Autodesk Inventor part; units mm, degrees
ref_plane "YZ Plane" through (0, 0, 0) normal (1, 0, 0) x (0, 1, 0)
ref_plane "XZ Plane" through (0, 0, 0) normal (0, 1, 0) x (-1, 0, 0)
ref_plane "XY Plane" through (0, 0, 0) normal (0, 0, 1) x (1, 0, 0)
sketch "スケッチ1" plane through (0, 0, 0) normal (0, 0, 1) x (1, 0, 0)
  line L0 (-30, 18) -> (30, 18)
  line L1 (30, 18) -> (30, -18)
  line L2 (30, -18) -> (-30, -18)
  line L3 (-30, -18) -> (-30, 18)
  line L4 (0, 0) -> (0, 18) construction
  line L5 (0, 0) -> (30, 0) construction
  dimension "d0" = 36
  dimension "d1" = 60
extrude "プレート1" add sketch "スケッチ1" along normal blind 3
sketch "スケッチ13" plane through (0, 0, 0) normal (0, 0, -1) x (-1, 0, 0)
  line L0 (0, 0) -> (30, 0) construction
  line L1 (30, -18) -> (30, 18)
  line L2 (-30, 18) -> (-30, -18)
  point P0 (23, 0)
  point P1 (-7, 0)
  dimension "d127" = 30
  dimension "d129" = 7
hole "穴10" at (-23, 0, 0) at (7, 0, 0) direction (0, 0, 1) diameter 7.9 depth 3
sketch "スケッチ15" plane through (0, 0, 0) normal (0, 0, -1) x (-1, 0, 0)
  circle A0 centre (-40, 0) radius 21
  line L0 (-30, -18) -> (-30, 18)
  point P0 (0, 0)
  dimension "d130" = 42
  dimension "d131" = 10
extrude "押し出し1" add sketch "スケッチ15" against normal up to surface (3 mm away)
fillet "フィレット1" radius 10 2 edges at (-30, 18, 1.5) (-30, -18, 1.5)
sketch "スケッチ16" plane through (0, 0, 0) normal (0, 0, -1) x (-1, 0, 0)
  arc A0 (-29.1833, 18) -> (-29.1833, -18) centre (-40, 0) ccw
  circle A1 centre (-40, 0) radius 14.5
  point P0 (0, 0)
  dimension "d134" = 29
extrude "押し出し2" cut sketch "スケッチ16" against normal up to surface (3 mm away)
sketch "スケッチ17" plane through (0, 0, 0) normal (0, 0, -1) x (-1, 0, 0)
  circle A0 centre (-40, 0) radius 14.5
  line L0 (-40, 0) -> (-61, 0) construction
  arc A1 (-29.1833, 18) -> (-29.1833, -18) centre (-40, 0) ccw
  point P0 (0, 0)
  point P1 (-58.5, 0)
  point P2 (-30.75, -16.0215)
  point P3 (-30.75, 16.0215)
  dimension "d137" = 18.5
  dimension "d140" = 360
hole "穴11" at (58.5, 0, 0) at (30.75, -16.0215, 0) at (30.75, 16.0215, 0) direction (0, 0, 1) diameter 2.7 depth 3
fillet "フィレット3" radius 50 2 edges at (29.1833, 18, 1.5) (29.1833, -18, 1.5)
equation "\"d125\" = Thickness"
equation "\"d147\" = Thickness"
equation "\"d2\" = Thickness"
equation "\"BendRadius\" = Thickness"
equation "\"BendReliefWidth\" = Thickness"
equation "\"BendReliefDepth\" = 0.5 * Thickness"
equation "\"CornerReliefSize\" = 4 * Thickness"
equation "\"MinimumRemnant\" = 2 * Thickness"
equation "\"TransitionRadius\" = BendRadius"
equation "\"JacobiRadiusSize\" = BendRadius"
equation "\"GapSize\" = Thickness"
properties part number "wrist_pitch_plate" material "アルミニウム 6061"
Geometry check sheet. Reference: the model listing, model coordinates, mm. A direction names the side the tool comes from. Round coordinates to 2 decimals unless told otherwise and drop trailing zeros. Loops run counter-clockwise (first coordinate to the right, second up) from the corner with the lowest first, then second, coordinate; pieces in that order, holes last. Notation, with made-up numbers: (-17, 17) -> (0, 17) arc R27 ccw to (0, 53) -> close; hole circle Ø6 at (-29, 33.25). An arc over 180 degrees is marked (long way). Answer as a JSON object with one key per item and string values. Group by question number.
Item 1: Thickness scan on line 1 along Y through (x, z) = (40, 2.7); line 2 along X through (y, z) = (1.5, 0.25); line 3 along X through (y, z) = (3, 1.1). Record the ranges inside material, lowest first.
Item 2: Release check for a two-part mould opening along X. For faces 1 (the face through (-19.144, -0.856, 1.521)), 2 (the face through (0, -18, 1)), 3 (the face through (26.948, 18.546, 1.479)) record: pulls with the +X half, pulls with the -X half, needs draft (parallel to the pull), parting line crosses it, or undercut.
Item 3: Cross-section at A-A, the plane x = 40. Record the cut outline in (y, z), plus the area to 3 significant figures.
Item 4: Set-up check for faces 4 (the face through (60.993, 0.548, 1.479)), 5 (the face through (0, 18, 1)): record each of +Z, -Z, +X, -X, +Y, -Y from which the full face is reachable in a straight line by a thin tool's end or side.
Item 5: Cross-section at C-C, the plane z = 1.4. Record the cut outline in (x, y), plus the area to 3 significant figures.
Item 6: Cross-section at B-B, the plane y = 0. Record the cut outline in (x, z), plus the area to 4 significant figures.
Item 7: Depth check by flat-ended pin: pin 1 Ø1.6 at (x, y) = (30.75, 16.02) entering from +Z; pin 2 Ø1.5 at (y, z) = (-16.5, 1.5) entering from -X. Enter the tip coordinate at first touch or a pass-through.
Item 8: Cross-section at D-D, the plane x = 7. Record the cut outline in (y, z), plus the area to 3 significant figures.
Determined:
{
 "1": {"line 1": "y = -21 to -14.5, 14.5 to 21", "line 2": "x = -30 to -26.65, -19.35 to 3.35, 10.65 to 25.58, 54.42 to 60.95", "line 3": "x = -30 to -25.57, -20.43 to 4.43, 9.57 to 25.81, 54.19 to 60.78"},
 "2": {"face 1": "undercut", "face 2": "needs draft", "face 3": "pulls with the -X half"},
 "3": {"outline": "(-21, 0) -> (-14.5, 0) -> (-14.5, 3) -> (-21, 3) -> close; (14.5, 0) -> (21, 0) -> (21, 3) -> (14.5, 3) -> close", "area": "39.0 mm²"},
 "4": {"face 4": "+Z, -Z", "face 5": "+Z, -Z, -X, +Y"},
 "5": {"outline": "(-30, -8) arc R10 ccw to (-20, -18) -> (19.58, -18) arc R50 cw to (33.96, -20.11) arc R21 ccw (long way) to (33.96, 20.11) arc R50 cw to (19.58, 18) -> (-20, 18) arc R10 ccw to (-30, 8) -> close; hole circle Ø7.9 at (-23, 0); hole circle Ø7.9 at (7, 0); hole circle Ø29 at (40, 0); hole circle Ø2.7 at (30.75, -16.02); hole circle Ø2.7 at (30.75, 16.02); hole circle Ø2.7 at (58.5, 0)", "area": "2,450 mm²"},
 "6": {"outline": "(-30, 0) -> (-26.95, 0) -> (-26.95, 3) -> (-30, 3) -> close; (-19.05, 0) -> (3.05, 0) -> (3.05, 3) -> (-19.05, 3) -> close; (10.95, 0) -> (25.5, 0) -> (25.5, 3) -> (10.95, 3) -> close; (54.5, 0) -> (57.15, 0) -> (57.15, 3) -> (54.5, 3) -> close; (59.85, 0) -> (61, 0) -> (61, 3) -> (59.85, 3) -> close", "area": "130.5 mm²"},
 "7": {"pin 1": "passes through", "pin 2": "stops at x = -26.32"},
 "8": {"outline": "(-18, 0) -> (-3.95, 0) -> (-3.95, 3) -> (-18, 3) -> close; (3.95, 0) -> (18, 0) -> (18, 3) -> (3.95, 3) -> close", "area": "84.3 mm²"}
}
